```python
from build123d import *

# Parameters (mm, degrees)
BOSS_EXTRUDE1_DEPTH = 2.8
CUT_EXTRUDE1_DEPTH  = 3.8
CUT_EXTRUDE2_DEPTH  = 3.8


with BuildPart() as part:
    # Sketch1 → Boss-Extrude1 (new body)
    with BuildSketch(Plane.XY):
        Polygon((-38.029024976, 83.602786166), (-38.029024976, -21.094016045), (34.914504121, -21.094016045), (34.914504121, 4.305983955), (19.039504121, 4.305983955), (-5.495011867, -2.268019791), (-28.504024976, 83.602786166), align=None)
    extrude(amount=BOSS_EXTRUDE1_DEPTH)

    # Sketch2 → Cut-Extrude1 (cut, through all)
    with BuildSketch(Plane.XY.offset(2.8)):
        Polygon((-19.264644206, -19.506516045), (-16.560051893, -18.781822719), (-17.284745219, -16.077230405), (-19.989337533, -16.801923732), align=None)
        Polygon((-28.646834591, 15.508295158), (-25.942242278, 16.232988484), (-35.324432663, 51.247799687), (-38.029024976, 61.341475615), (-38.029024976, 50.523106361), align=None)
    extrude(amount=-CUT_EXTRUDE1_DEPTH, mode=Mode.SUBTRACT)

    # Sketch3 → Cut-Extrude2 (cut, through all)
    with BuildSketch(Plane.XY.offset(2.8)):
        Polygon((28.814978037, -19.506516045), (31.51957035, -18.781822719), (30.794877024, -16.077230405), (28.09028471, -16.801923732), align=None)
        Polygon((23.58624935, 0.007365071), (26.290841664, 0.732058397), (25.333211197, 4.305983955), (22.434437892, 4.305983955), (22.628618883, 3.581290628), align=None)
    extrude(amount=-CUT_EXTRUDE2_DEPTH, mode=Mode.SUBTRACT)


solid = part.part
```
The model under review builds one solid part; all positions refer to its coordinate system, in mm. A direction names the side the tool comes from. Give positions to 0.01 mm unless a question says otherwise; leave off trailing zeros. Write each loop counter-clockwise with the first axis right and the second up, starting at its lowest first coordinate (ties: lowest second). Pieces come first, ordered by that corner, then holes. Notation, with made-up numbers: (83.5, 32) -> (103.5, 32) arc R21 ccw to (103.5, 65) -> close; hole circle Ø3 at (46.25, 69.5). An arc over 180 degrees is marked (long way). Answer in a Markdown table with one row per item.
1) Add section B-B on y = 30.5. State the section outline as (x, z) points, plus the area to 3 significant figures.
Worked answers:
| item | result |
|---|---|
| outline | (-38.03, 0) -> (-32.66, 0) -> (-32.66, 2.8) -> (-38.03, 2.8) -> close; (-29.77, 0) -> (-14.28, 0) -> (-14.28, 2.8) -> (-29.77, 2.8) -> close |
| area | 58.4 mm² |
2) Add section C-C on x = -27. State the section outline as (y, z) points.
Worked answers:
| item | result |
|---|---|
| outline | (-21.09, 0) -> (15.95, 0) -> (15.95, 2.8) -> (-21.09, 2.8) -> close; (20.18, 0) -> (77.99, 0) -> (77.99, 2.8) -> (20.18, 2.8) -> close |
3) Mouldability with a two-part tool opening along Y and no side actions: class faces 6 (the flat face through (30, 4.306, 1)), 7 (the flat face through (-10, 9, 0)), 8 (the flat face through (31.162, -17.448, 1.42)), 9 (the flat face through (-2, -21.094, 1)) as +Y half, -Y half, draft (parallel to the pull), parting line (faces both ways), or undercut.
Worked answers:
| item | result |
|---|---|
| face 6 | +Y half |
| face 7 | draft |
| face 8 | undercut |
| face 9 | -Y half |
4) Clearance check with flat-ended pins moving along their axes: P1, Ø0.8, axis at x = 29.5, z = 1.5, coming from the +Y side; P2, Ø1.5, axis at y = 61, z = 2.5, coming from the +X side. State where each tip first meets the part, or that it passes through.
Worked answers:
| item | result |
|---|---|
| P1 | y = 4.31 |
| P2 | x = -22.25 |
5) Add section A-A on z = 2.1. State the section outline as (x, y) points, plus the area to 3 significant figures.
Worked answers:
| item | result |
|---|---|
| outline | (-38.03, -21.09) -> (34.91, -21.09) -> (34.91, 4.31) -> (25.33, 4.31) -> (26.29, 0.73) -> (23.59, 0.01) -> (22.43, 4.31) -> (19.04, 4.31) -> (-5.5, -2.27) -> (-28.5, 83.6) -> (-38.03, 83.6) -> (-38.03, 61.34) -> (-25.94, 16.23) -> (-28.65, 15.51) -> (-38.03, 50.52) -> close; hole (-19.99, -16.8) -> (-19.26, -19.51) -> (-16.56, -18.78) -> (-17.28, -16.08) -> close; hole (28.09, -16.8) -> (28.81, -19.51) -> (31.52, -18.78) -> (30.79, -16.08) -> close |
| area | 3,220 mm² |
6) Add section D-D on y = 60. State the section outline as (x, z) points.
Worked answers:
| item | result |
|---|---|
| outline | (-37.67, 0) -> (-22.18, 0) -> (-22.18, 2.8) -> (-37.67, 2.8) -> close |
7) Tool access review of faces 1 (the flat face through (6.944, 1.065, 1.38)), 2 (the flat face through (-38.029, 73, 1)), 3 (the flat face through (21, 4.306, 1)), 4 (the flat face through (-33, 83.603, 1)), 5 (the flat face through (29.462, -16.435, 1.42)): name each direction out of +Z, -Z, +X, -X, +Y, -Y from which nothing blocks a thin tool from reaching the whole face with its end or side.
Worked answers:
| item | result |
|---|---|
| face 1 | +Z, -Z, +Y |
| face 2 | +Z, -Z, -X, +Y, -Y |
| face 3 | +Z, -Z, +X, +Y |
| face 4 | +Z, -Z, +X, -X, +Y |
| face 5 | +Z, -Z |
8) For L1, parallel to Y at x = 13.5, z = 2.15; L2, parallel to X at y = 40, z = 0.5; L3, parallel to X at y = 17.5, z = 0.4, list the stretches that pass through material, from the lowest coordinate up. Write a range as [from, to].
Worked answers:
| item | result |
|---|---|
| L1 | [-21.09, 2.82] |
| L2 | [-38.03, -35.21], [-32.31, -16.82] |
| L3 | [-38.03, -29.18], [-26.28, -10.79] |
